from build123d import *

# Parameters (mm, degrees)
F0_R     = 12.4
F1_DEPTH = 6
F2_W     = 5
F2_H     = 5
F3_DEPTH = 50
F4_R     = 0.75
F5_DEPTH = 60


with BuildPart() as f1:
    # F0 (on Front) → F1 (new body)
    with BuildSketch(Plane.XZ):
        Circle(F0_R)
    extrude(amount=F1_DEPTH)

    # F2 (on face) → F3 (join)
    with BuildSketch(Plane.XZ.offset(6)):
        Rectangle(F2_W, F2_H)
    extrude(amount=F3_DEPTH)

    # F4 (on face) → F5 (cut)
    with BuildSketch(Plane(origin=(0, 0, 0), x_dir=(-1, 0, 0), z_dir=(0, 1, 0))):
        with Locations((0, 2.5)):
            Circle(F4_R)
    extrude(amount=-F5_DEPTH, mode=Mode.SUBTRACT)


solid = f1.part
The model under review builds one solid part; all positions refer to its coordinate system, in mm. A direction names the side the tool comes from. Coordinates: 2 decimals unless noted, no trailing zeros. Order: outer loops, then holes, each group sorted by start corner. A loop starts at its lowest first (then second) coordinate and runs counter-clockwise, first axis right, second up. Notation, with made-up numbers: (-32.75, 16.5) -> (24.25, 16.5) arc R7 ccw to (24.25, 29.5) -> close; hole circle Ø7 at (47.5, 30). An arc over 180 degrees is marked (long way). Answer in a Markdown table with one row per item.
(1) Machinability: for faces 5 (the flat face through (-2.5, -31, 0)), 6 (the flat face through (-2, -31, 2.5)), 7 (the flat face through (2.5, -31, 0)), which of the approach directions +Z, -Z, +X, -X, +Y, -Y give a long, thin tool a straight path to every point of the face, cutting with its end or side? Answer none if there is none.
Answers:
| item | result |
|---|---|
| face 5 | +Z, -Z, -X, -Y |
| face 6 | +Z, +X, -X, -Y |
| face 7 | +Z, -Z, +X, -Y |
(2) The part is to be moulded in two halves that separate along Z. For faces 1 (the cylindrical face through (-0.346, -27.608, 1.835)), 2 (the flat face through (2, -31, 2.5)), 3 (the cylindrical face through (5.72, -2.96, -11)), 4 (the flat face through (0, -6, -3)), say which applies: +Z half, -Z half, draft (parallel to the pull), parting line (faces both ways), or undercut.
Answers:
| item | result |
|---|---|
| face 1 | undercut |
| face 2 | +Z half |
| face 3 | parting line |
| face 4 | draft |
(3) Consider section B-B (z = 0). Write out the cut boundary in (x, y), plus the area to 3 significant figures.
Answers:
| item | result |
|---|---|
| outline | (-12.4, -6) -> (-2.5, -6) -> (-2.5, -56) -> (2.5, -56) -> (2.5, -6) -> (12.4, -6) -> (12.4, 0) -> (-12.4, 0) -> close |
| area | 399 mm² |
(4) Consider section A-A (x = 0). Write out the cut boundary in (y, z), plus the area to 3 significant figures.
Answers:
| item | result |
|---|---|
| outline | (-56, -2.5) -> (-6, -2.5) -> (-6, -12.4) -> (0, -12.4) -> (0, 1.75) -> (-56, 1.75) -> close; (-6, 3.25) -> (0, 3.25) -> (0, 12.4) -> (-6, 12.4) -> close |
| area | 352 mm² |
(5) Insertion check: pin 1 (1.5 mm diameter, centred on y = -40, z = 0.5, fed in from -X); pin 2 (2 mm diameter, centred on x = -4.5, y = -50, fed in from +Z); pin 3 (2.5 mm diameter, centred on y = -25, z = 0, fed in from +X); pin 4 (0.5 mm diameter, centred on x = 2, y = -22.5, fed in from +Z). Each pin has a flat end and moves straight along its axis. Give the tip position at first contact, or say it passes through.
Answers:
| item | result |
|---|---|
| pin 1 | x = -2.5 |
| pin 2 | through |
| pin 3 | x = 2.5 |
| pin 4 | z = 2.5 |
(6) Consider section D-D (x = 6). Write out the cut boundary in (y, z).
Answers:
| item | result |
|---|---|
| outline | (-6, -10.85) -> (0, -10.85) -> (0, 10.85) -> (-6, 10.85) -> close |
(7) Consider section C-C (y = -38.5). Write out the cut boundary in (x, z).
Answers:
| item | result |
|---|---|
| outline | (-2.5, -2.5) -> (2.5, -2.5) -> (2.5, 2.5) -> (0.75, 2.5) arc R0.75 cw to (-0.75, 2.5) -> (-2.5, 2.5) -> close |
(8) Wall thickness on line 1 along Y through (x, z) = (7.5, -3.5); line 2 along Z through (x, y) = (0, -22); line 3 along Z through (x, y) = (-0.25, -2.5): over which ranges is each line inside the solid? List them lowest first.
Answers:
| item | result |
|---|---|
| line 1 | -6 to 0 |
| line 2 | -2.5 to 1.75 |
| line 3 | -12.4 to 1.79, 3.21 to 12.4 |
